```python
from build123d import *

# Parameters (mm, degrees)
F1_DEPTH = 1200


with BuildPart() as f1:
    # F0 (on Front) → F1 (new body, symmetric)
    with BuildSketch(Plane.XZ):
        with BuildLine():
            Line((0, 14), (0, 0))
            Line((0, 0), (180, 0))
            Line((180, 0), (180, 14))
            Line((180, 14), (109.25, 14))
            ThreePointArc((109.25, 14), (98.643398, 18.393398), (94.25, 29))
            Line((94.25, 29), (94.25, 151))
            ThreePointArc((94.25, 151), (98.643398, 161.606602), (109.25, 166))
            Line((109.25, 166), (180, 166))
            Line((180, 166), (180, 180))
            Line((180, 180), (0, 180))
            Line((0, 180), (0, 166))
            Line((0, 166), (70.75, 166))
            ThreePointArc((70.75, 166), (81.356602, 161.606602), (85.75, 151))
            Line((85.75, 151), (85.75, 29))
            ThreePointArc((85.75, 29), (81.356602, 18.393398), (70.75, 14))
            Line((70.75, 14), (0, 14))
        make_face()
    extrude(amount=F1_DEPTH, both=True)


solid = f1.part
```
Input: part model. Units: mm. Frame: model coordinates. A direction names the side the tool comes from. Round coordinates to 2 decimals unless told otherwise and drop trailing zeros. Loops run counter-clockwise (first coordinate to the right, second up) from the corner with the lowest first, then second, coordinate; pieces in that order, holes last.
1) Section query A-A on x = 131.5. Return the cut outline in (y, z).
Ans:
outline: (-1200, 0) - (1200, 0) - (1200, 14) - (-1200, 14) - close; (-1200, 166) - (1200, 166) - (1200, 180) - (-1200, 180) - close
2) Pull-direction query (Z, two-part tool) for faces 4 (the flat face through (144, -17, 166)), 5 (the flat face through (91, -17, 180)), 6 (the flat face through (90, -1200, 90)); classes: released by +Z, released by -Z, zero draft, split by the parting line, or undercut.
Ans:
face 4: undercut
face 5: released by +Z
face 6: zero draft
3) Section query C-C on z = 102. Return the cut outline in (x, y).
Ans:
outline: (85.75, -1200) - (94.25, -1200) - (94.25, 1200) - (85.75, 1200) - close
4) Section query B-B on y = -904.5. Return the cut outline in (x, z), plus the area to 3 significant figures.
Ans:
outline: (0, 0) - (180, 0) - (180, 14) - (109.25, 14) arc R15 cw to (94.25, 29) - (94.25, 151) arc R15 cw to (109.25, 166) - (180, 166) - (180, 180) - (0, 180) - (0, 166) - (70.75, 166) arc R15 cw to (85.75, 151) - (85.75, 29) arc R15 cw to (70.75, 14) - (0, 14) - close
area: 6,530 mm2
5) Pin query (flat end, axial travel): pin 1 (2 mm diameter, centred on y = 466.5, z = 133, fed in from -X); pin 2 (1.5 mm diameter, centred on y = 327, z = 43.5, fed in from +X); pin 3 (2 mm diameter, centred on y = 554.5, z = 29, fed in from -X). Return the tip coordinate at first contact, or that it passes through.
Ans:
pin 1: stops at x = 85.75
pin 2: stops at x = 94.25
pin 3: stops at x = 85.72
6) Material intervals for line 1 (Z direction, x = 69.5, y = -437.5); line 2 (Z direction, x = 72.5, y = -327.5); line 3 (X direction, y = -174.5, z = 74), sorted ascending.
Ans:
line 1: z = 0 to 14, 166 to 180
line 2: z = 0 to 14.1, 165.9 to 180
line 3: x = 85.75 to 94.25
7) Set-up query: faces 1 (the flat face through (90, 1200, 90)), 2 (the flat face through (85.75, -17, 91)), 3 (the flat face through (145, -17, 14)). Return all of +Z, -Z, +X, -X, +Y, -Y with unobstructed straight access to the full face (end or side cutting, diameter ignored); none if empty.
Ans:
face 1: +Z, -Z, +X, -X, +Y
face 2: -X, +Y, -Y
face 3: +X, +Y, -Y
